```python
from build123d import *

# Parameters (mm, degrees)
SKETCH1_W               = 48.4
SKETCH1_H               = 50.8
BOSS_EXTRUDE1_DEPTH     = 85.62
CUT_EXTRUDE1_DEPTH      = 49.4
CUT_EXTRUDE2_DEPTH      = 70
SKETCH5_R               = 5.5
CUT_EXTRUDE3_DEPTH      = 80
SKETCH6_R               = 3.25
CUT_EXTRUDE4_DEPTH      = 6.62
CUT_EXTRUDE5_DEPTH      = 3
CUT_EXTRUDE5_DEPTH_BACK = 3
CUT_EXTRUDE6_REACH      = 35.4
SKETCH8_W               = 6
SKETCH8_H               = 10
CUT_EXTRUDE7_REACH      = 52.8
SKETCH4_R               = 3.25
FILLET1_R               = 3.81


with BuildPart() as part:
    # Sketch1 → Boss-Extrude1 (new body)
    with BuildSketch(Plane(origin=(0, 0, 0), x_dir=(0, 1, 0), z_dir=(0, 0, 1))):
        with Locations((24.2, 25.4)):
            Rectangle(SKETCH1_W, SKETCH1_H)
    extrude(amount=BOSS_EXTRUDE1_DEPTH)

    # Sketch2 → Cut-Extrude1 (cut, through all)
    with BuildSketch(Plane(origin=(0, 48.4, 0), x_dir=(-1, 0, 0), z_dir=(0, 1, 0))):
        Polygon((26.8, 85.62), (0, 25.62), (0, 85.62), align=None)
    extrude(amount=-CUT_EXTRUDE1_DEPTH, mode=Mode.SUBTRACT)

    # Sketch3 → Cut-Extrude2 (cut)
    with BuildSketch(Plane(origin=(0, 0, 0), x_dir=(1, 0, 0), z_dir=(0, 0, -1))):
        Polygon((-43.8, 0), (-43.8, -3), (-46.8, -3), (-46.8, -15), (-30.8, -15), (-30.8, -3), (-33.8, -3), (-33.8, 0), align=None)
    extrude(amount=-CUT_EXTRUDE2_DEPTH, mode=Mode.SUBTRACT)

    # Sketch5 → Cut-Extrude3 (cut)
    with BuildSketch(Plane.XY.offset(85.62)):
        with Locations((-12.7, 10.3)):
            Circle(SKETCH5_R)
        with Locations((-12.7, 35.7)):
            Circle(SKETCH5_R)
    extrude(amount=-CUT_EXTRUDE3_DEPTH, mode=Mode.SUBTRACT)

    # Sketch6 → Cut-Extrude4 (cut, through all)
    with BuildSketch(Plane.XY.offset(5.62)):
        with Locations((-12.7, 35.7)):
            Circle(SKETCH6_R)
        with Locations((-12.7, 10.3)):
            Circle(SKETCH6_R)
    extrude(amount=-CUT_EXTRUDE4_DEPTH, mode=Mode.SUBTRACT)

    # Sketch7 → Cut-Extrude5 (cut, two sides)
    with BuildSketch(Plane.ZY.offset(38.8)) as cut_extrude5_sk:
        Polygon((35.6, 43.773502692), (30.6, 40.886751346), (30.6, 35.113248654), (35.6, 32.226497308), (40.6, 35.113248654), (40.6, 40.886751346), align=None)
    extrude(amount=CUT_EXTRUDE5_DEPTH, mode=Mode.SUBTRACT)
    extrude(cut_extrude5_sk.sketch, amount=-CUT_EXTRUDE5_DEPTH_BACK, mode=Mode.SUBTRACT)

    # Sketch8 → Cut-Extrude6 (cut, up to next)
    with BuildSketch(Plane.XZ.offset(-15), mode=Mode.PRIVATE) as cut_extrude6_sk1:
        with Locations((-38.8, 35.6)):
            Rectangle(SKETCH8_W, SKETCH8_H)
    cut_extrude6_tool1 = extrude(cut_extrude6_sk1.sketch, amount=-CUT_EXTRUDE6_REACH, mode=Mode.PRIVATE) & part.part
    add(cut_extrude6_tool1.solids().sort_by_distance((-38.8, 15, 35.6))[0], mode=Mode.SUBTRACT)

    # Sketch4 → Cut-Extrude7 (cut, up to next)
    with BuildSketch(Plane(origin=(-50.8, 0, 0), x_dir=(0, -1, 0), z_dir=(-1, 0, 0)), mode=Mode.PRIVATE) as cut_extrude7_sk1:
        with Locations((-38, 35.6)):
            Circle(SKETCH4_R)
    cut_extrude7_tool1 = extrude(cut_extrude7_sk1.sketch, amount=-CUT_EXTRUDE7_REACH, mode=Mode.PRIVATE) & part.part
    add(cut_extrude7_tool1.solids().sort_by_distance((-50.8, 38, 35.6))[0], mode=Mode.SUBTRACT)

    # Fillet1
    fillet1_edges = [part.edges().sort_by_distance(p)[0] for p in [
        (-38.8, 48.4, 85.62),
        (0, 48.4, 12.81),
        (-26.8, 24.2, 85.62),
        (0, 24.2, 25.62),
        (-13.4, 48.4, 55.62),
        (-50.8, 48.4, 42.81),
    ]]
    fillet(fillet1_edges, radius=FILLET1_R)


solid = part.part
```
CAD build for the part. Positions are in the model's coordinates, mm. A direction names the side the tool comes from. Coordinates: 2 decimals unless noted, no trailing zeros. Order: outer loops, then holes, each group sorted by start corner. A loop starts at its lowest first (then second) coordinate and runs counter-clockwise, first axis right, second up.
(1) Saw through at A-A, the plane y = 25.5. Write the cut outline in (x, z), and give its area (3 significant figures).
Solution:
outline: (-50.8, 0) - (0, 0) - (0, 24.81) arc R3.81 ccw to (-0.33, 26.36) - (-25.79, 83.36) arc R3.81 ccw to (-29.27, 85.62) - (-50.8, 85.62) - close; hole (-41.8, 30.6) - (-35.8, 30.6) - (-35.8, 40.6) - (-41.8, 40.6) - close
area: 3,480 mm2
(2) Saw through at C-C, the plane y = 10.3. Write the cut outline in (x, z).
Solution:
outline: (-50.8, 0) - (-46.8, 0) - (-46.8, 70) - (-30.8, 70) - (-30.8, 0) - (-15.95, 0) - (-15.95, 5.62) - (-18.2, 5.62) - (-18.2, 66.37) - (-25.79, 83.36) arc R3.81 ccw to (-29.27, 85.62) - (-50.8, 85.62) - close; (-9.45, 0) - (0, 0) - (0, 24.81) arc R3.81 ccw to (-0.33, 26.36) - (-7.2, 41.74) - (-7.2, 5.62) - (-9.45, 5.62) - close
(3) Mould opens along Z. For faces 1 (the face through (-10, 33, 5.62)), 2 (the face through (-46.36, 34.9, 36.58)), 3 (the face through (-32, 3, 35)) say: released by +Z, released by -Z, zero draft, split by the parting line, or undercut.
Solution:
face 1: released by +Z
face 2: undercut
face 3: zero draft
(4) Pin check, flat tips, straight feed: pin 1 Ø12 at (x, y) = (-21, 22) entering from +Z; pin 2 Ø10 at (x, y) = (-12.7, 35.7) entering from +Z; pin 3 Ø4 at (y, z) = (31, 33) entering from +X. Stop position of each tip, or through.
Solution:
pin 1: stops at z = 84.87
pin 2: stops at z = 5.62
pin 3: stops at x = -2.4
(5) Drill centre lines: L1, parallel to Y at x = -12.7, z = 3.5; L2, parallel to Y at x = -12.7, z = 40.5; L3, parallel to X at y = 4.5, z = 20. Where is each one in solid material? Low to high.
Solution:
L1: y = 0 to 7.05, 13.55 to 32.45, 38.95 to 48.4
L2: y = 0 to 4.8, 15.8 to 30.2, 41.2 to 48.4
L3: x = -50.8 to -46.8, -30.8 to 0
(6) Which spindle directions (+Z, -Z, +X, -X, +Y, -Y) get a long thin tool onto all of the face, cutting with end or side? Do faces 4 (the face through (-10, 8, 5.62)), 5 (the face through (-39, 28, 30.6)), 6 (the face through (-40, 22, 85.62)), 7 (the face through (-30.8, 9, 35)), 8 (the face through (-26, 24, 0)). Say none if no direction does.
Solution:
face 4: +Z
face 5: -Y
face 6: +Z, +X, -X, +Y, -Y
face 7: -Z
face 8: -Z, +X, -X, +Y, -Y
(7) Saw through at B-B, the plane y = 35.7. Write the cut outline in (x, z).
Solution:
outline: (-50.8, 0) - (-15.95, 0) - (-15.95, 5.62) - (-18.2, 5.62) - (-18.2, 66.37) - (-25.79, 83.36) arc R3.81 ccw to (-29.27, 85.62) - (-50.8, 85.62) - (-50.8, 37.9) - (-41.8, 37.9) - (-41.8, 40.6) - (-35.8, 40.6) - (-35.8, 30.6) - (-41.8, 30.6) - (-41.8, 33.3) - (-50.8, 33.3) - close; (-9.45, 0) - (0, 0) - (0, 24.81) arc R3.81 ccw to (-0.33, 26.36) - (-7.2, 41.74) - (-7.2, 5.62) - (-9.45, 5.62) - close
